Here's how the part is built. I have some questions about the finished solid (model axes, mm). A direction names the side the tool comes from. Coordinates: 2 decimals unless noted, no trailing zeros. Loops run counter-clockwise (first coordinate to the right, second up) from the corner with the lowest first, then second, coordinate; pieces in that order, holes last. Notation, with made-up numbers: (88, 31.25) - (136, 31.25) arc R13 cw to (136, 56.25) - close; hole circle Ø6 at (67, 20.25). An arc over 180 degrees is marked (long way). Use a Markdown table: item, result.
```python
from build123d import *

# Parameters (mm, degrees)
SKETCH1_R               = 11.811
BOSS_EXTRUDE1_DEPTH     = 50.8
BOSS_EXTRUDE2_DEPTH     = 2.399999772
SKETCH5_R               = 3.81
SKETCH5_W               = 12.7
SKETCH5_H               = 5.08
SKETCH5_W_2             = 15.24
SKETCH5_H_2             = 23.622
CUT_EXTRUDE3_DEPTH      = 3.81
SKETCH8_W               = 53.199999772
SKETCH8_H               = 53.199999772
BOSS_EXTRUDE3_DEPTH     = 12.7
CUT_EXTRUDE5_DEPTH      = 99.371995605
CUT_EXTRUDE5_DEPTH_BACK = 3.81
SKETCH6_R               = 4.7625
FILLET1_R               = 2.54


with BuildPart() as part:
    # Sketch1 → Boss-Extrude1 (new body)
    with BuildSketch(Plane(origin=(0, 0, 0), x_dir=(0, 0, -1), z_dir=(1, 0, 0))):
        with BuildLine():
            Line((-63.5, 14.210999772), (63.5, 14.210999772))
            ThreePointArc((63.5, 14.210999772), (77.710999772, 0), (63.5, -14.210999772))
            Line((63.5, -14.210999772), (-63.5, -14.210999772))
            ThreePointArc((-63.5, -14.210999772), (-77.710999772, 0), (-63.5, 14.210999772))
        make_face()
        with Locations((-63.5, 0)):
            Circle(SKETCH1_R, mode=Mode.SUBTRACT)
        with Locations((63.5, 0)):
            Circle(SKETCH1_R, mode=Mode.SUBTRACT)
        with BuildLine():
            Line((-55.597292014, 11.811), (55.597292014, 11.811))
            ThreePointArc((55.597292014, 11.811), (49.289000228, 0), (55.597292014, -11.811))
            Line((55.597292014, -11.811), (-55.597292014, -11.811))
            ThreePointArc((-55.597292014, -11.811), (-49.289000228, 0), (-55.597292014, 11.811))
        make_face(mode=Mode.SUBTRACT)
    extrude(amount=BOSS_EXTRUDE1_DEPTH)

    # Sketch2 → Boss-Extrude2 (add)
    with BuildSketch(Plane(origin=(50.8, 0, 0), x_dir=(0, 0, -1), z_dir=(1, 0, 0))):
        with BuildLine():
            Line((-63.5, -14.210999772), (63.5, -14.210999772))
            ThreePointArc((63.5, -14.210999772), (77.710999772, 0), (63.5, 14.210999772))
            Line((63.5, 14.210999772), (-63.5, 14.210999772))
            ThreePointArc((-63.5, 14.210999772), (-77.710999772, 0), (-63.5, -14.210999772))
        make_face()
    extrude(amount=BOSS_EXTRUDE2_DEPTH)

    # Sketch5 → Cut-Extrude3 (cut)
    with BuildSketch(Plane.ZY.offset(-50.8)):
        with Locations((41.669000228, 4.191)):
            Circle(SKETCH5_R)
        with Locations((-42.939000228, 6.731)):
            Rectangle(SKETCH5_W, SKETCH5_H)
        Rectangle(SKETCH5_W_2, SKETCH5_H_2)
    extrude(amount=-CUT_EXTRUDE3_DEPTH, mode=Mode.SUBTRACT)

    # Sketch8 → Boss-Extrude3 (add)
    with BuildSketch(Plane(origin=(0, 14.210999772, 0), x_dir=(1, 0, 0), z_dir=(0, 1, 0))):
        with Locations((26.599999886, 0)):
            Rectangle(SKETCH8_W, SKETCH8_H)
    extrude(amount=BOSS_EXTRUDE3_DEPTH)

    # Sketch6 → Cut-Extrude5 (cut, two sides: drawn at the far end of the back side and taken through both)
    with BuildSketch(Plane(origin=(0, 14.210999772, 0), x_dir=(1, 0, 0), z_dir=(0, 1, 0)).offset(-CUT_EXTRUDE5_DEPTH_BACK)):
        with Locations(Location((26.599999886, 0, 0), (0, 0, 270))):
            Circle(SKETCH6_R)
    extrude(amount=CUT_EXTRUDE5_DEPTH + CUT_EXTRUDE5_DEPTH_BACK, mode=Mode.SUBTRACT)

    # Fillet1
    fillet1_edges = [part.edges().sort_by_distance(p)[0] for p in [
        (26.599999886, 14.210999772, 26.599999886),
        (26.599999886, 14.210999772, -26.599999886),
    ]]
    fillet(fillet1_edges, radius=FILLET1_R)


solid = part.part
```
Q1. I want a section at C-C, the plane y = 21. Write out the boundary of the cut face in (x, z) (1 decimal).
Check values:
| item | result |
|---|---|
| outline | (0, -26.6) - (53.2, -26.6) - (53.2, 26.6) - (0, 26.6) - close; hole circle Ø9.5 at (26.6, 0) |
Q2. I want a section at B-B, the plane z = 0. Write out the boundary of the cut face in (x, y).
Check values:
| item | result |
|---|---|
| outline | (0, -14.21) - (53.2, -14.21) - (53.2, -11.81) - (0, -11.81) - close; (0, 11.81) - (21.84, 11.81) - (21.84, 26.91) - (0, 26.91) - close; (31.36, 11.81) - (53.2, 11.81) - (53.2, 26.91) - (31.36, 26.91) - close |
Q3. I want a section at A-A, the plane x = 38. Write out the boundary of the cut face in (y, z), then the cut area to 3 significant figures.
Check values:
| item | result |
|---|---|
| outline | (-14.21, -63.5) arc R14.21 ccw to (14.21, -63.5) - (14.21, -29.14) arc R2.54 cw to (16.75, -26.6) - (26.91, -26.6) - (26.91, 26.6) - (16.75, 26.6) arc R2.54 cw to (14.21, 29.14) - (14.21, 63.5) arc R14.21 ccw to (-14.21, 63.5) - close; hole circle Ø23.62 at (0, -63.5); hole (-11.81, -55.6) arc R14.21 cw to (11.81, -55.6) - (11.81, 55.6) arc R14.21 cw to (-11.81, 55.6) - close; hole circle Ø23.62 at (0, 63.5) |
| area | 1,630 mm^2 |
Q4. Which directions (+Z, -Z, +X, -X, +Y, -Y) give clear straight access to the entire face, cutting with the end or side of a thin tool? Please do faces 4 (the face through (50.8, 0, -63)), 5 (the face through (26, 14.211, 46)), 6 (the face through (26, 14.211, -47)).
Check values:
| item | result |
|---|---|
| face 4 | -X |
| face 5 | +Z, +X, -X, +Y |
| face 6 | -Z, +X, -X, +Y |
Q5. Will these pins go through, and if not, where does the flat tip stop? P1, Ø17, axis at x = 29, z = -51.5, coming from the +Y side; P2, Ø1, axis at y = 13.5, z = 35.5, coming from the -X side; P3, Ø11, axis at x = 33.5, y = 21.5, coming from the -Z side; P4, Ø1.9, axis at x = 52.5, y = -3, coming from the +Z side.
Check values:
| item | result |
|---|---|
| P1 | y = 14.21 |
| P2 | x = 0 |
| P3 | z = -26.71 |
| P4 | z = 77.56 |
Q6. I want a section at D-D, the plane x = 26.6. Write out the boundary of the cut face in (y, z).
Check values:
| item | result |
|---|---|
| outline | (-14.21, -63.5) arc R14.21 ccw to (14.21, -63.5) - (14.21, -29.14) arc R2.54 cw to (16.75, -26.6) - (26.91, -26.6) - (26.91, -4.76) - (11.81, -4.76) - (11.81, -55.6) arc R14.21 ccw to (-11.81, -55.6) - (-11.81, 55.6) arc R14.21 ccw to (11.81, 55.6) - (11.81, 4.76) - (26.91, 4.76) - (26.91, 26.6) - (16.75, 26.6) arc R2.54 cw to (14.21, 29.14) - (14.21, 63.5) arc R14.21 ccw to (-14.21, 63.5) - close; hole circle Ø23.62 at (0, -63.5); hole circle Ø23.62 at (0, 63.5) |
Q7. If we mould it in two halves opening along Z, with no side actions, what happens to faces 1 (the face through (26, 22, -26.6)), 2 (the face through (26, 22, 26.6)), 3 (the face through (31.32, 19.26, -0.62))? For each: pulls with the +Z half, pulls with the -Z half, needs draft (parallel to the pull), parting line crosses it, or undercut.
Check values:
| item | result |
|---|---|
| face 1 | pulls with the -Z half |
| face 2 | pulls with the +Z half |
| face 3 | undercut |
Q8. Please list where these lines run through material, in increasing order: L1, parallel to Y at x = 28, z = -63.5; L2, parallel to Y at x = 22, z = 3.5; L3, parallel to Z at x = 26.6, y = 17.5. Write a range as from..to.
Check values:
| item | result |
|---|---|
| L1 | -14.21..-11.81, 11.81..14.21 |
| L2 | -14.21..-11.81, 11.81..26.91 |
| L3 | -26.6..-4.76, 4.76..26.6 |
